Could you check a few things on this model? Use its own coordinates, in mm. A direction names the side the tool comes from. Coordinates: 2 decimals unless noted, no trailing zeros. Loops run counter-clockwise (first coordinate to the right, second up) from the corner with the lowest first, then second, coordinate; pieces in that order, holes last. Notation, with made-up numbers: (3.25, 5) - (41.25, 5) arc R19 cw to (41.25, 39) - close; hole circle Ø4 at (64, 17). An arc over 180 degrees is marked (long way). Use CSV: the item, a comma, the result in double quotes.
from build123d import *

# Parameters (mm, degrees)
SKETCH1_W             = 43
SKETCH1_H             = 43
BOSS_EXTRUDE1_DEPTH   = 4
SKETCH2_W             = 49
SKETCH2_H             = 49
SKETCH2_W_2           = 43
SKETCH2_H_2           = 43
BOSS_EXTRUDE2_DEPTH   = 16
FILLET1_R             = 10
SKETCH3_W             = 49
SKETCH3_H             = 49
SKETCH3_R             = 12.5
BOSS_EXTRUDE3_DEPTH   = 4
F_4_0MM_DOWEL_HOLE1_D = 4
CHAMFER1_SIZE         = 3
CHAMFER3_SIZE         = 0.5
CHAMFER4_SIZE         = 1
SKETCH8_W             = 38.715759924
SKETCH8_H             = 37.056710796
BOSS_EXTRUDE4_DEPTH   = 0.2
SKETCH9_R             = 12.5
CUT_EXTRUDE2_DEPTH    = 49.757460968
SKETCH10_R            = 2
CUT_EXTRUDE3_DEPTH    = 49.757460968


with BuildPart() as part:
    # Sketch1 → Boss-Extrude1 (new body)
    with BuildSketch(Plane(origin=(0, 0, 0), x_dir=(1, 0, 0), z_dir=(0, 1, 0))):
        with BuildLine():
            Line((-24.5, 24.5), (-19.330127019, 24.5))
            ThreePointArc((-19.330127019, 24.5), (-21.614378278, 32.291287847), (-15, 37))
            Line((-15, 37), (15, 37))
            ThreePointArc((15, 37), (21.614378278, 32.291287847), (19.330127019, 24.5))
            Line((19.330127019, 24.5), (24.5, 24.5))
            Line((24.5, 24.5), (24.5, 6.437196595))
            Line((24.5, 6.437196595), (24.5, -24.5))
            Line((24.5, -24.5), (19.330127019, -24.5))
            ThreePointArc((19.330127019, -24.5), (21.614378278, -32.291287847), (15, -37))
            Line((15, -37), (-15, -37))
            ThreePointArc((-15, -37), (-21.614378278, -32.291287847), (-19.330127019, -24.5))
            Line((-19.330127019, -24.5), (-24.5, -24.5))
            Line((-24.5, -24.5), (-24.5, 6.437196595))
            Line((-24.5, 6.437196595), (-24.5, 24.5))
        make_face()
        Rectangle(SKETCH1_W, SKETCH1_H, mode=Mode.SUBTRACT)
        with BuildLine():
            Line((15, 27), (-15, 27))
            ThreePointArc((-15, 27), (-18, 30), (-15, 33))
            Line((-15, 33), (15, 33))
            ThreePointArc((15, 33), (18, 30), (15, 27))
        make_face(mode=Mode.SUBTRACT)
        with BuildLine():
            Line((-15, -27), (15, -27))
            ThreePointArc((15, -27), (18, -30), (15, -33))
            Line((15, -33), (-15, -33))
            ThreePointArc((-15, -33), (-18, -30), (-15, -27))
        make_face(mode=Mode.SUBTRACT)
    extrude(amount=BOSS_EXTRUDE1_DEPTH)

    # Sketch2 → Boss-Extrude2 (add)
    with BuildSketch(Plane(origin=(0, 4, 0), x_dir=(1, 0, 0), z_dir=(0, 1, 0))):
        Rectangle(SKETCH2_W, SKETCH2_H)
        Rectangle(SKETCH2_W_2, SKETCH2_H_2, mode=Mode.SUBTRACT)
    extrude(amount=BOSS_EXTRUDE2_DEPTH)

    # Fillet1
    # the kernel refuses this fillet: 10 mm, written as the material it adds along each edge
    with BuildSketch(Plane(origin=(19.330127019, 0, 24.5), x_dir=(0.405761244184207, 0, 0.913979109563279), z_dir=(0, 1, 0))) as fillet1_piece_1:
        with BuildLine():
            CenterArc((11.211042432, 8.841903543), FILLET1_R, 204.310084353, 37.841965765)
            Line((2.097734093, 4.725155904), (1.915467926, 4.642820951))
            ThreePointArc((1.915467926, 4.642820951), (0.866071225, 2.443730201), (-0.182795822, 0.081152249))
            Line((-0.182795822, 0.081152249), (0.093425354, -0.176838071))
            ThreePointArc((0.093425354, -0.176838071), (3.269887376, 0.61066752), (6.446349398, -0.176838071))
            Line((6.446349398, -0.176838071), (6.539774752, 0))
        make_face()
    extrude(amount=4)
    with BuildSketch(Plane(origin=(19.330127019, 0, -24.5), x_dir=(1, 0, 0), z_dir=(0, 1, 0))) as fillet1_piece_2:
        with BuildLine():
            CenterArc((12.630321653, 6.658956796), FILLET1_R, 183.909110465, 37.841965765)
            Line((2.65358714, 5.977217504), (2.45405245, 5.963582719))
            ThreePointArc((2.45405245, 5.963582719), (1.884930926, 2.74082354), (-0.123717915, 0.157142857))
            Line((-0.123717915, 0.157142857), (0, -0.2))
            ThreePointArc((0, -0.2), (2.584936491, -0.2), (5.020664008, -0.133179136))
            Line((5.020664008, -0.133179136), (5.169872981, 0))
        make_face()
    extrude(amount=4)
    with BuildSketch(Plane(origin=(-19.330127019, 0, -24.5), x_dir=(-1, 0, 0), z_dir=(0, 1, 0))) as fillet1_piece_3:
        with BuildLine():
            CenterArc((12.630321653, -6.658956796), FILLET1_R, 138.24892377, 37.841965765)
            Line((2.65358714, -5.977217504), (2.45405245, -5.963582719))
            ThreePointArc((2.45405245, -5.963582719), (1.884930926, -2.74082354), (-0.123717915, -0.157142857))
            Line((-0.123717915, -0.157142857), (0, 0.2))
            ThreePointArc((0, 0.2), (2.584936491, 0.2), (5.020664008, 0.133179136))
            Line((5.020664008, 0.133179136), (5.169872981, 0))
        make_face()
    extrude(amount=4)
    with BuildSketch(Plane(origin=(-19.330127019, 0, 24.5), x_dir=(-0.40576124418420745, 0, 0.9139791095632787), z_dir=(0, 1, 0))) as fillet1_piece_4:
        with BuildLine():
            CenterArc((11.211042432, -8.841903543), FILLET1_R, 117.847949882, 37.841965765)
            Line((2.097734093, -4.725155904), (1.915467926, -4.642820951))
            ThreePointArc((1.915467926, -4.642820951), (0.866071225, -2.443730201), (-0.182795822, -0.081152249))
            Line((-0.182795822, -0.081152249), (0.093425354, 0.176838071))
            ThreePointArc((0.093425354, 0.176838071), (3.269887376, -0.61066752), (6.446349398, 0.176838071))
            Line((6.446349398, 0.176838071), (6.539774752, 0))
        make_face()
    extrude(amount=4)

    # Sketch3 → Boss-Extrude3 (add)
    with BuildSketch(Plane(origin=(0, 20, 0), x_dir=(1, 0, 0), z_dir=(0, 1, 0))):
        Rectangle(SKETCH3_W, SKETCH3_H)
        with Locations(Location((0, 0, 0), (0, 0, 270))):
            Circle(SKETCH3_R, mode=Mode.SUBTRACT)
    extrude(amount=BOSS_EXTRUDE3_DEPTH)

    # Ø4.0mm Dowel Hole1 (through all)
    with Locations(Plane(origin=(0, 24, 0), x_dir=(1, 0, 0), z_dir=(0, 1, 0))):
        with Locations((15.5, 15.5), (-15.5, 15.5), (-15.5, -15.5), (15.5, -15.5)):
            Hole(F_4_0MM_DOWEL_HOLE1_D / 2)

    # Chamfer1
    chamfer1_edges = [part.edges().sort_by_distance(p)[0] for p in [
        (24.5, 24, 0),
        (0, 24, -24.5),
        (-24.5, 24, 0),
        (0, 24, 24.5),
        (-24.5, 14, 24.5),
        (-24.5, 14, -24.5),
        (24.5, 14, -24.5),
        (24.5, 14, 24.5),
        (-21.5, 10, -21.5),
        (-21.5, 10, 21.5),
        (21.5, 10, 21.5),
        (21.5, 10, -21.5),
    ]]
    chamfer(chamfer1_edges, length=CHAMFER1_SIZE)

    # Chamfer3
    chamfer3_edges = [part.edges().sort_by_distance(p)[0] for p in [
        (0, 20, -12.5),
        (0, 24, -12.5),
        (17.5, 24, 15.5),
        (-13.5, 24, 15.5),
        (-13.5, 24, -15.5),
        (17.5, 24, -15.5),
    ]]
    chamfer(chamfer3_edges, length=CHAMFER3_SIZE)

    # Chamfer4
    chamfer4_edges = [part.edges().sort_by_distance(p)[0] for p in [
        (-19.778047586, 4, 35.115687761),
        (19.778047586, 4, -35.115687761),
        (0, 4, -37),
        (-22.743853768, 4, 27.278959583),
        (22.743853768, 4, 27.278959583),
        (22.743853768, 4, -27.278959583),
        (-22.743853768, 4, -27.278959583),
        (-19.778047586, 4, -35.115687761),
        (18, 4, 30),
        (0, 4, 33),
        (-18, 4, 30),
        (18, 4, -30),
        (0, 4, -27),
        (-18, 4, -30),
        (0, 4, -33),
        (0, 4, 37),
        (19.778047586, 4, 35.115687761),
        (0, 4, 27),
    ]]
    chamfer(chamfer4_edges, length=CHAMFER4_SIZE)

    # Sketch8 → Boss-Extrude4 (add)
    with BuildSketch(Plane.XZ.offset(-20)):
        Rectangle(SKETCH8_W, SKETCH8_H)
    extrude(amount=-BOSS_EXTRUDE4_DEPTH)

    # Sketch9 → Cut-Extrude2 (cut, through all)
    with BuildSketch(Plane(origin=(0, 20.2, 0), x_dir=(1, 0, 0), z_dir=(0, 1, 0))):
        with Locations(Location((0, 0, 0), (0, 0, 90))):
            Circle(SKETCH9_R)
    extrude(amount=-CUT_EXTRUDE2_DEPTH, mode=Mode.SUBTRACT)

    # Sketch10 → Cut-Extrude3 (cut, through all)
    with BuildSketch(Plane(origin=(0, 20.2, 0), x_dir=(1, 0, 0), z_dir=(0, 1, 0))):
        with Locations(Location((-15.5, 15.5, 0), (0, 0, 90))):
            Circle(SKETCH10_R)
        with Locations(Location((-15.5, -15.5, 0), (0, 0, 90))):
            Circle(SKETCH10_R)
        with Locations(Location((15.5, -15.5, 0), (0, 0, 90))):
            Circle(SKETCH10_R)
        with Locations(Location((15.5, 15.5, 0), (0, 0, 90))):
            Circle(SKETCH10_R)
    extrude(amount=-CUT_EXTRUDE3_DEPTH, mode=Mode.SUBTRACT)


solid = part.part
(1) Suppose I cut it at C-C (x = -11). State how many separate pieces and enclosed holes the cut face has, plus the area to 3 significant figures.
Computed:
separate pieces,"4"
enclosed holes,"0"
area,"308 mm²"
(2) Suppose I cut it at A-A (z = -15.5). Write out the boundary of the cut face in (x, y), plus the area to 4 significant figures.
Computed:
outline,"(-24.5, 0) - (-21.5, 0) - (-21.5, 20) - (-17.5, 20) - (-17.5, 23.5) - (-18, 24) - (-21.5, 24) - (-24.5, 21) - close; (-13.5, 20) - (13.5, 20) - (13.5, 23.5) - (13, 24) - (-13, 24) - (-13.5, 23.5) - close; (17.5, 20) - (21.5, 20) - (21.5, 0) - (24.5, 0) - (24.5, 21) - (21.5, 24) - (18, 24) - (17.5, 23.5) - close"
area,"274.5 mm²"
(3) Please list where these lines run through material, in increasing order: line 1 (X direction, y = 20.1, z = 0); line 2 (Z direction, x = -2.5, y = 11); line 3 (X direction, y = 20.75, z = 15.5).
Computed:
line 1,"x = -24.5 to -12.5, 12.5 to 24.5"
line 2,"z = -24.5 to -21.5, 21.5 to 24.5"
line 3,"x = -24.5 to -17.5, -13.5 to 13.5, 17.5 to 24.5"
(4) Thinking about a two-plate mould opening in Z: for faces 1 (the face through (0, 1, 37)), 2 (the face through (18, 1, -30)), 3 (the face through (-19.832, 1.479, -35.065)), which applies, +Z half, -Z half, draft (parallel to the pull), parting line (faces both ways), or undercut?
Computed:
face 1,"+Z half"
face 2,"undercut"
face 3,"-Z half"
(5) Will these pins go through, and if not, where does the flat tip stop? pin 1 (8.5 mm diameter, centred on x = 6, y = 14, fed in from -Z); pin 2 (5 mm diameter, centred on x = 5, y = 16, fed in from +Z); pin 3 (13 mm diameter, centred on x = 6, z = 8, fed in from -Y).
Computed:
pin 1,"stops at z = -24.5"
pin 2,"stops at z = 24.5"
pin 3,"stops at y = 20"
(6) Which directions (+Z, -Z, +X, -X, +Y, -Y) give clear straight access to the entire face, cutting with the end or side of a thin tool? Please do faces 4 (the face through (0, 12, 24.5)), 5 (the face through (0, 12, -24.5)), 6 (the face through (23, 22.5, 0.3)), 7 (the face through (-18, 1, 30)), 8 (the face through (20, 10, 20)).
Computed:
face 4,"+Z, +X, -X, +Y"
face 5,"-Z, +X, -X, +Y"
face 6,"+Z, -Z, +X, +Y"
face 7,"+Y, -Y"
face 8,"-Y"
(7) Suppose I cut it at B-B (y = 13). Write out the boundary of the cut face in (x, z).
Computed:
outline,"(-24.5, -21.5) - (-21.5, -24.5) - (21.5, -24.5) - (24.5, -21.5) - (24.5, 21.5) - (21.5, 24.5) - (-21.5, 24.5) - (-24.5, 21.5) - close; hole (-21.5, -18.5) - (-18.5, -21.5) - (18.5, -21.5) - (21.5, -18.5) - (21.5, 18.5) - (18.5, 21.5) - (-18.5, 21.5) - (-21.5, 18.5) - close"
